Answer from the drawing. Dimensions are ordinates in mm from the lowest x, y and z of the part. A direction names the side the tool comes from. Give positions to 0.01 mm unless a question says otherwise; leave off trailing zeros. Write each loop counter-clockwise with the first axis right and the second up, starting at its lowest first coordinate (ties: lowest second). Pieces come first, ordered by that corner, then holes. Notation, with made-up numbers: (74, 9.5) -> (98, 9.5) arc R20 cw to (98, 47.5) -> close; hole circle Ø11 at (49.25, -35.5). An arc over 180 degrees is marked (long way). Write item = value, one per line.
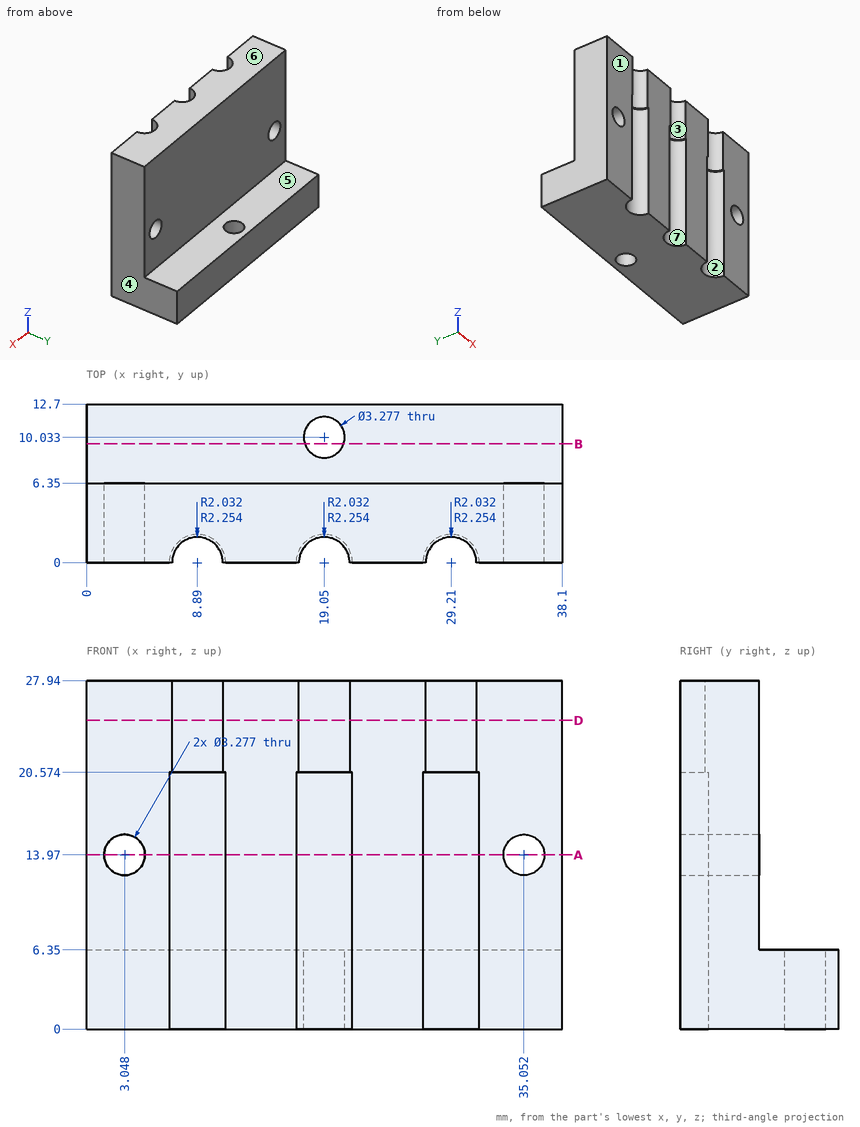
(1) A tool of negligible diameter and unlimited length cuts with its end or side. For the marked faces 5, 6 and 7, from which of +Z, -Z, +X, -X, +Y, -Y can it reach the whole face along a straight path? Write none if from no direction.
Checks:
face_5 = +Z, +X, -X, +Y
face_6 = +Z, +X, -X, +Y, -Y
face_7 = -Z, -Y
(2) The part is cut by section D-D on z = 24.75. Determine the outline of the cut face in (x, y).
Checks:
outline = (0, 0) -> (6.86, 0) arc R2.03 cw to (10.92, 0) -> (17.02, 0) arc R2.03 cw to (21.08, 0) -> (27.18, 0) arc R2.03 cw to (31.24, 0) -> (38.1, 0) -> (38.1, 6.35) -> (0, 6.35) -> close
(3) The part is cut by section A-A on z = 13.97. Count the separate pieces of the cut face and the enclosed holes in it, plus the area to 3 significant figures.
Checks:
separate_pieces = 3
enclosed_holes = 0
area = 176 mm²
(4) For a pull along X with two mould halves and no side action, classify the marked faces 1, 2, 3 and 4 as released by +X, released by -X, zero draft, split by the parting line, or undercut.
Checks:
face_1 = zero draft
face_2 = undercut
face_3 = undercut
face_4 = released by +X
(5) The part is cut by section B-B on y = 9.5. Determine the outline of the cut face in (x, z).
Checks:
outline = (0, 0) -> (17.5, 0) -> (17.5, 6.35) -> (0, 6.35) -> close; (20.6, 0) -> (38.1, 0) -> (38.1, 6.35) -> (20.6, 6.35) -> close
(6) Consider L1, parallel to X at y = 3.5, z = 13.97; L2, parallel to Y at x = 19.05, z = 2 (1 decimal); L3, parallel to X at y = 1, z = 17.5. Determine where each line is inside the solid, lowest interval first.
Checks:
L1 = 0 to 1.41, 4.69 to 33.41, 36.69 to 38.1
L2 = 2.3 to 8.4, 11.7 to 12.7
L3 = 0 to 6.87, 10.91 to 17.03, 21.07 to 27.19, 31.23 to 38.1
(7) Given P1, Ø12, axis at x = 33.5, z = 14.5, coming from the +Y side, flat-ended and moving along its own axis, determine where the tip first touches the part or whether it passes through.
Checks:
P1 = 6.35
